Read the model definition and answer for the solid it produces. Units are mm, in the model's axes. Face numbers are marked on the shaded views. A direction names the side the tool comes from. Coordinates: 2 decimals unless noted, no trailing zeros. Write each loop counter-clockwise with the first axis right and the second up, starting at its lowest first coordinate (ties: lowest second). Pieces come first, ordered by that corner, then holes. Notation, with made-up numbers: (-25.75, 48.5) -> (-15.75, 48.5) arc R17 cw to (-15.75, 76.5) -> close; hole circle Ø11 at (42.25, -34.75). An arc over 180 degrees is marked (long way). Write item = value, one per line. Start each with the question number.
1) A tool of negligible diameter and unlimited length cuts with its end or side. For the marked faces 4 and 5, from which of +Z, -Z, +X, -X, +Y, -Y can it reach the whole face along a straight path? Write none if from no direction.
2) Section A-A (z = 45) is taken. Count the separate pieces of the cut face and the enclosed holes in it, plus the area to 3 significant figures.
3) For a pull along X with two mould halves and no side action, classify the marked faces 1, 2 and 3 as released by +X, released by -X, zero draft, split by the parting line, or undercut.
4) Section D-D (x = 0) is taken. Determine the outline of the cut face in (y, z) (3 decimals).
5) Flat-ended cylindrical pins translate along their axes: pin 1 Ø17 at (x, y) = (33.34, 0) entering from -Z; pin 2 Ø5 at (x, z) = (-39, 11.5) entering from +Y; pin 3 Ø5 at (x, y) = (-7.5, 33.5) entering from +Z; pin 4 Ø1.5 at (x, y) = (4.5, 39.5) entering from +Z. Find the tip coordinate at first contact, or state that the pin passes through.
6) Section B-B (x = 33.5) is taken. Determine the outline of the cut face in (y, z), plus the area to 3 significant figures.
7) Find the intervals of material crossed by line 1 along Y through (x, z) = (34, 33); line 2 along X through (y, z) = (3, 6.5); line 3 along Y through (x, z) = (17.5, 11.5), in increasing order. Write a range as from..to.
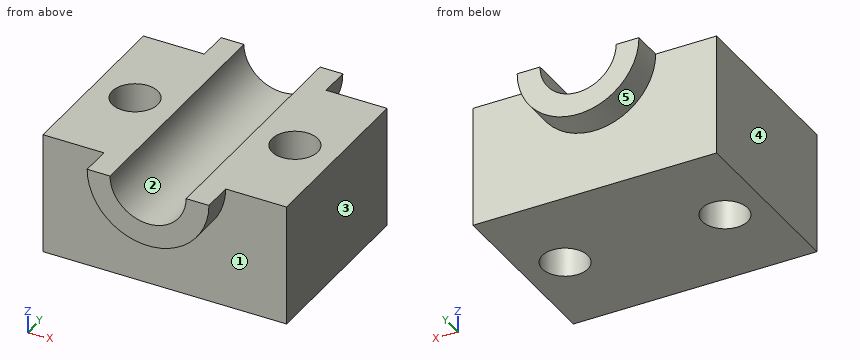
from build123d import *

# Parameters (mm, degrees)
F0_W          = 101.6
F0_H          = 76.2
F1_DEPTH      = 50.8
F3_DEPTH      = 12.7
F3_DEPTH_BACK = 88.9
F4_R          = 15.875
F5_DEPTH      = 122.936
F6_R          = 9.525
F7_DEPTH      = 135.636
F8_R          = 9.525
F9_DEPTH      = 98.298


with BuildPart() as f1:
    # F0 (on Top) → F1 (new body)
    with BuildSketch(Plane.XY):
        Rectangle(F0_W, F0_H)
    extrude(amount=F1_DEPTH)

    # F2 (on face) → F3 (join, two sides)
    with BuildSketch(Plane.XZ.offset(38.1)) as f3_sk:
        with BuildLine():
            Line((25.4, 50.8), (-25.4, 50.8))
            ThreePointArc((-25.4, 50.8), (0, 25.4), (25.4, 50.8))
        make_face()
    extrude(amount=F3_DEPTH)
    extrude(f3_sk.sketch, amount=-F3_DEPTH_BACK)

    # F4 (on face) → F5 (cut)
    with BuildSketch(Plane.XZ.offset(50.8)):
        with Locations((0, 50.8)):
            Circle(F4_R)
    extrude(amount=-F5_DEPTH, mode=Mode.SUBTRACT)

    # F6 (on face) → F7 (cut)
    with BuildSketch(Plane.XY.offset(50.8)):
        with Locations((-33.3375, 0)):
            Circle(F6_R)
    extrude(amount=-F7_DEPTH, mode=Mode.SUBTRACT)

    # F8 (on face) → F9 (cut)
    with BuildSketch(Plane.XY.offset(50.8)):
        with Locations((33.3375, 0)):
            Circle(F8_R)
    extrude(amount=-F9_DEPTH, mode=Mode.SUBTRACT)


solid = f1.part
Answer key:
q1.face_4 = +Z, -Z, -X, +Y, -Y
q1.face_5 = -Z, +Y
q2.separate_pieces = 2
q2.enclosed_holes = 2
q2.area = 5,430 mm^2
q3.face_1 = zero draft
q3.face_2 = undercut
q3.face_3 = released by +X
q4.outline = (-50.8, 25.4) -> (-38.1, 25.4) -> (-38.1, 0) -> (38.1, 0) -> (38.1, 25.4) -> (50.8, 25.4) -> (50.8, 34.925) -> (-50.8, 34.925) -> close
q5.pin_1 = through
q5.pin_2 = 38.1
q5.pin_3 = 38.47
q5.pin_4 = 35.82
q6.outline = (-38.1, 0) -> (-9.52, 0) -> (-9.52, 50.8) -> (-38.1, 50.8) -> close; (9.52, 0) -> (38.1, 0) -> (38.1, 50.8) -> (9.52, 50.8) -> close
q6.area = 2,900 mm^2
q7.line_1 = -38.1..-9.5, 9.5..38.1
q7.line_2 = -50.8..-42.38, -24.3..24.3, 42.38..50.8
q7.line_3 = -38.1..38.1
